```python
from build123d import *

# Parameters (mm, degrees)
SKETCH_1_W          = 150
SKETCH_1_H          = 140
EXTRUDE_1_DEPTH     = 3
SKETCH_3_R          = 1.75
CUT_EXTRUDE_1_DEPTH = 10
SKETCH_4_R          = 1.35
CUT_EXTRUDE_2_DEPTH = 10
SKETCH_5_R          = 1.6
CUT_EXTRUDE_3_DEPTH = 10
FILLET_1_R          = 5


with BuildPart() as part:
    # 草图1 → 凸台-拉伸1 (new body)
    with BuildSketch(Plane.XY):
        Rectangle(SKETCH_1_W, SKETCH_1_H)
    extrude(amount=EXTRUDE_1_DEPTH)

    # 草图3 → 切除-拉伸1 (cut)
    with BuildSketch(Plane.XY.offset(3)):
        with Locations((25, 40)):
            Circle(SKETCH_3_R)
        with Locations((-39, 40)):
            Circle(SKETCH_3_R)
        with Locations((25, 8.5)):
            Circle(SKETCH_3_R)
        with Locations((-39, 8.5)):
            Circle(SKETCH_3_R)
    extrude(amount=-CUT_EXTRUDE_1_DEPTH, mode=Mode.SUBTRACT)

    # 草图4 → 切除-拉伸2 (cut)
    with BuildSketch(Plane.XY.offset(3)):
        with Locations((25, -20)):
            Circle(SKETCH_4_R)
        with Locations((-11, -20)):
            Circle(SKETCH_4_R)
        with Locations((-11, -56)):
            Circle(SKETCH_4_R)
        with Locations((25, -56)):
            Circle(SKETCH_4_R)
    extrude(amount=-CUT_EXTRUDE_2_DEPTH, mode=Mode.SUBTRACT)

    # 草图5 → 切除-拉伸3 (cut)
    with BuildSketch(Plane.XY.offset(3)):
        with Locations((65, 60)):
            Circle(SKETCH_5_R)
        with Locations((-65, 60)):
            Circle(SKETCH_5_R)
        with Locations((65, -60)):
            Circle(SKETCH_5_R)
    extrude(amount=-CUT_EXTRUDE_3_DEPTH, mode=Mode.SUBTRACT)

    # 圆角1
    fillet_1_edges = [part.edges().sort_by_distance(p)[0] for p in [
        (75, -70, 1.5),
        (-75, -70, 1.5),
        (-75, 70, 1.5),
        (75, 70, 1.5),
    ]]
    fillet(fillet_1_edges, radius=FILLET_1_R)


solid = part.part
```
Work out the finished part from the listing and answer in its coordinate system (mm). Give positions to 0.01 mm unless a question says otherwise; leave off trailing zeros. Loops run counter-clockwise (first coordinate to the right, second up) from the corner with the lowest first, then second, coordinate; pieces in that order, holes last. Notation, with made-up numbers: (9.25, 45) - (65.25, 45) arc R22 cw to (65.25, 81) - close; hole circle Ø9 at (-16.5, 51.5). An arc over 180 degrees is marked (long way). Use CSV: the item, a comma, the result in double quotes. Start each with the question number.
(1) This flat-tipped pin is pushed along its axis until it touches: pin 1 (2.5 mm diameter, centred on x = -11, y = -56, fed in from +Z). Where does it stop, or does it pass through?
(2) Find the intervals of material crossed by L1, parallel to Y at x = -11, z = 0.95; L2, parallel to Y at x = 65, z = 2, in increasing order.
(3) Find section A-A, the plane y = 8.5. Determine the outline of the cut face in (x, z).
(4) Determine the mould class of faces 1 (the face through (-74, -68, 2)), 2 (the face through (73, 69, 2)), 3 (the face through (66.526, 60.481, 1.521)) for opening direction Y: released by +Y, released by -Y, zero draft, split by the parting line, or undercut.
Results found:
1,pin 1,"through"
2,L1,"-70 to -57.35, -54.65 to -21.35, -18.65 to 70"
2,L2,"-70 to -61.6, -58.4 to 58.4, 61.6 to 70"
3,outline,"(-75, 0) - (-40.75, 0) - (-40.75, 3) - (-75, 3) - close; (-37.25, 0) - (23.25, 0) - (23.25, 3) - (-37.25, 3) - close; (26.75, 0) - (75, 0) - (75, 3) - (26.75, 3) - close"
4,face 1,"released by -Y"
4,face 2,"released by +Y"
4,face 3,"undercut"
